```python
from build123d import *

# Parameters (mm, degrees)
BOSS_1_DEPTH    = 5
BOSS_2_DEPTH    = 4.5
S_CYL3_R        = 9.5
BOSS_3_DEPTH    = 3.2
BOSS_4_DEPTH    = 4.5
S_HOLE5_R       = 3.5
HOLE_5_DEPTH    = 4.7
S_HOLE6_R       = 1.7
HOLE_6_DEPTH    = 4.7
S_HOLE7_R       = 1.7
HOLE_7_DEPTH    = 4.7
S_HOLE8_R       = 1.7
HOLE_8_DEPTH    = 4.7
S_HOLE9_R       = 1.7
HOLE_9_DEPTH    = 4.7
S_HOLE10_R      = 3.2
HOLE_10_DEPTH   = 1.6
S_HOLE11_R      = 3.2
HOLE_11_DEPTH   = 1.6
S_HOLE12_R      = 3.2
HOLE_12_DEPTH   = 1.6
S_HOLE13_R      = 3.2
HOLE_13_DEPTH   = 1.6
S_HOLE14_R      = 3.5
HOLE_14_DEPTH   = 7.9
S_HOLE15_R      = 1.7
HOLE_15_DEPTH   = 7.9
S_HOLE16_R      = 1.7
HOLE_16_DEPTH   = 7.9
S_HOLE17_R      = 1.7
HOLE_17_DEPTH   = 7.9
S_HOLE18_R      = 1.7
HOLE_18_DEPTH   = 7.9
S_HOLE19_R      = 3.2
HOLE_19_DEPTH   = 2.1
S_HOLE20_R      = 3.2
HOLE_20_DEPTH   = 2.1
S_HOLE21_R      = 3.2
HOLE_21_DEPTH   = 2.1
S_HOLE22_R      = 3.2
HOLE_22_DEPTH   = 2.1
S_CUT23_W       = 1
S_CUT23_H       = 6.8
POCKET_23_DEPTH = 10
S_HOLE24_R      = 6
HOLE_24_DEPTH   = 5.2
S_HOLE25_R      = 6
HOLE_25_DEPTH   = 5.2
S_HOLE26_R      = 6
HOLE_26_DEPTH   = 5.2
S_CUT27_W       = 1.1
S_CUT27_H       = 4.5
POCKET_27_DEPTH = 16
S_CUT28_W       = 1.1
S_CUT28_H       = 4.5
POCKET_28_DEPTH = 16


with BuildPart() as part:
    # S_prism1 → Boss_1 (new body)
    with BuildSketch(Plane.XY.offset(-33)):
        Polygon((56, -21), (56, 21), (42, 35), (-58, 35), (-68, 25), (-68, -25), (-58, -35), (42, -35), align=None)
    extrude(amount=BOSS_1_DEPTH)

    # S_prism2 → Boss_2 (add)
    with BuildSketch(Plane(origin=(-22, 0, 0), x_dir=(0, 0, -1), z_dir=(1, 0, 0))):
        with BuildLine():
            Line((28.5, -16), (28.5, 16))
            Line((28.5, 16), (-1.0301, 13.8653))
            ThreePointArc((-1.0301, 13.8653), (-9.544808445, 9.785590923), (-13, 0.9989))
            Line((-13, 0.9989), (-13, -0.9989))
            ThreePointArc((-13, -0.9989), (-9.544808445, -9.785590923), (-1.0301, -13.8653))
            Line((-1.0301, -13.8653), (28.5, -16))
        make_face()
    extrude(amount=BOSS_2_DEPTH)



with BuildPart() as body_2:
    # S_cyl3 → Boss_3 (new body)
    with BuildSketch(Plane(origin=(-61.75, 0, 0), x_dir=(0, 0, -1), z_dir=(1, 0, 0))):
        Circle(S_CYL3_R)
    extrude(amount=BOSS_3_DEPTH)


with BuildPart() as part_1:
    add(part.part)

    add(body_2.part)  # Boss_4 merges body 2
    # S_prism4 → Boss_4 (add)
    with BuildSketch(Plane(origin=(-66.25, 0, 0), x_dir=(0, 0, -1), z_dir=(1, 0, 0))):
        with BuildLine():
            Line((28.5, -16), (28.5, 16))
            Line((28.5, 16), (-1.0301, 13.8653))
            ThreePointArc((-1.0301, 13.8653), (-9.544808445, 9.785590923), (-13, 0.9989))
            Line((-13, 0.9989), (-13, -0.9989))
            ThreePointArc((-13, -0.9989), (-9.544808445, -9.785590923), (-1.0301, -13.8653))
            Line((-1.0301, -13.8653), (28.5, -16))
        make_face()
    extrude(amount=BOSS_4_DEPTH)

    # S_hole5 → Hole_5 (cut)
    with BuildSketch(Plane(origin=(-22.1, 0, 0), x_dir=(0, 0, -1), z_dir=(1, 0, 0))):
        Circle(S_HOLE5_R)
    extrude(amount=HOLE_5_DEPTH, mode=Mode.SUBTRACT)

    # S_hole6 → Hole_6 (cut)
    with BuildSketch(Plane(origin=(-22.1, 0, 0), x_dir=(0, 0, -1), z_dir=(1, 0, 0))):
        with Locations((0, 7)):
            Circle(S_HOLE6_R)
    extrude(amount=HOLE_6_DEPTH, mode=Mode.SUBTRACT)

    # S_hole7 → Hole_7 (cut)
    with BuildSketch(Plane(origin=(-22.1, 0, 0), x_dir=(0, 0, -1), z_dir=(1, 0, 0))):
        with Locations((-7, 0)):
            Circle(S_HOLE7_R)
    extrude(amount=HOLE_7_DEPTH, mode=Mode.SUBTRACT)

    # S_hole8 → Hole_8 (cut)
    with BuildSketch(Plane(origin=(-22.1, 0, 0), x_dir=(0, 0, -1), z_dir=(1, 0, 0))):
        with Locations((0, -7)):
            Circle(S_HOLE8_R)
    extrude(amount=HOLE_8_DEPTH, mode=Mode.SUBTRACT)

    # S_hole9 → Hole_9 (cut)
    with BuildSketch(Plane(origin=(-22.1, 0, 0), x_dir=(0, 0, -1), z_dir=(1, 0, 0))):
        with Locations((7, 0)):
            Circle(S_HOLE9_R)
    extrude(amount=HOLE_9_DEPTH, mode=Mode.SUBTRACT)

    # S_hole10 → Hole_10 (cut)
    with BuildSketch(Plane(origin=(-19, 0, 0), x_dir=(0, 0, -1), z_dir=(1, 0, 0))):
        with Locations((0, 7)):
            Circle(S_HOLE10_R)
    extrude(amount=HOLE_10_DEPTH, mode=Mode.SUBTRACT)

    # S_hole11 → Hole_11 (cut)
    with BuildSketch(Plane(origin=(-19, 0, 0), x_dir=(0, 0, -1), z_dir=(1, 0, 0))):
        with Locations((-7, 0)):
            Circle(S_HOLE11_R)
    extrude(amount=HOLE_11_DEPTH, mode=Mode.SUBTRACT)

    # S_hole12 → Hole_12 (cut)
    with BuildSketch(Plane(origin=(-19, 0, 0), x_dir=(0, 0, -1), z_dir=(1, 0, 0))):
        with Locations((0, -7)):
            Circle(S_HOLE12_R)
    extrude(amount=HOLE_12_DEPTH, mode=Mode.SUBTRACT)

    # S_hole13 → Hole_13 (cut)
    with BuildSketch(Plane(origin=(-19, 0, 0), x_dir=(0, 0, -1), z_dir=(1, 0, 0))):
        with Locations((7, 0)):
            Circle(S_HOLE13_R)
    extrude(amount=HOLE_13_DEPTH, mode=Mode.SUBTRACT)

    # S_hole14 → Hole_14 (cut)
    with BuildSketch(Plane(origin=(-66.35, 0, 0), x_dir=(0, 0, -1), z_dir=(1, 0, 0))):
        Circle(S_HOLE14_R)
    extrude(amount=HOLE_14_DEPTH, mode=Mode.SUBTRACT)

    # S_hole15 → Hole_15 (cut)
    with BuildSketch(Plane(origin=(-66.35, 0, 0), x_dir=(0, 0, -1), z_dir=(1, 0, 0))):
        with Locations((0, 7)):
            Circle(S_HOLE15_R)
    extrude(amount=HOLE_15_DEPTH, mode=Mode.SUBTRACT)

    # S_hole16 → Hole_16 (cut)
    with BuildSketch(Plane(origin=(-66.35, 0, 0), x_dir=(0, 0, -1), z_dir=(1, 0, 0))):
        with Locations((-7, 0)):
            Circle(S_HOLE16_R)
    extrude(amount=HOLE_16_DEPTH, mode=Mode.SUBTRACT)

    # S_hole17 → Hole_17 (cut)
    with BuildSketch(Plane(origin=(-66.35, 0, 0), x_dir=(0, 0, -1), z_dir=(1, 0, 0))):
        with Locations((0, -7)):
            Circle(S_HOLE17_R)
    extrude(amount=HOLE_17_DEPTH, mode=Mode.SUBTRACT)

    # S_hole18 → Hole_18 (cut)
    with BuildSketch(Plane(origin=(-66.35, 0, 0), x_dir=(0, 0, -1), z_dir=(1, 0, 0))):
        with Locations((7, 0)):
            Circle(S_HOLE18_R)
    extrude(amount=HOLE_18_DEPTH, mode=Mode.SUBTRACT)

    # S_hole19 → Hole_19 (cut)
    with BuildSketch(Plane(origin=(-66.35, 0, 0), x_dir=(0, 0, -1), z_dir=(1, 0, 0))):
        with Locations((0, 7)):
            Circle(S_HOLE19_R)
    extrude(amount=HOLE_19_DEPTH, mode=Mode.SUBTRACT)

    # S_hole20 → Hole_20 (cut)
    with BuildSketch(Plane(origin=(-66.35, 0, 0), x_dir=(0, 0, -1), z_dir=(1, 0, 0))):
        with Locations((-7, 0)):
            Circle(S_HOLE20_R)
    extrude(amount=HOLE_20_DEPTH, mode=Mode.SUBTRACT)

    # S_hole21 → Hole_21 (cut)
    with BuildSketch(Plane(origin=(-66.35, 0, 0), x_dir=(0, 0, -1), z_dir=(1, 0, 0))):
        with Locations((0, -7)):
            Circle(S_HOLE21_R)
    extrude(amount=HOLE_21_DEPTH, mode=Mode.SUBTRACT)

    # S_hole22 → Hole_22 (cut)
    with BuildSketch(Plane(origin=(-66.35, 0, 0), x_dir=(0, 0, -1), z_dir=(1, 0, 0))):
        with Locations((7, 0)):
            Circle(S_HOLE22_R)
    extrude(amount=HOLE_22_DEPTH, mode=Mode.SUBTRACT)

    # S_cut23 → Pocket_23 (cut)
    with BuildSketch(Plane.XY):
        with Locations((-58.95, 0)):
            Rectangle(S_CUT23_W, S_CUT23_H)
    extrude(amount=POCKET_23_DEPTH, mode=Mode.SUBTRACT)

    # S_hole24 → Hole_24 (cut)
    with BuildSketch(Plane.XY.offset(-33.1)):
        with Locations((-40, 0)):
            Circle(S_HOLE24_R)
    extrude(amount=HOLE_24_DEPTH, mode=Mode.SUBTRACT)

    # S_hole25 → Hole_25 (cut)
    with BuildSketch(Plane.XY.offset(-33.1)):
        with Locations((14, 0)):
            Circle(S_HOLE25_R)
    extrude(amount=HOLE_25_DEPTH, mode=Mode.SUBTRACT)

    # S_hole26 → Hole_26 (cut)
    with BuildSketch(Plane.XY.offset(-33.1)):
        with Locations((36, 0)):
            Circle(S_HOLE26_R)
    extrude(amount=HOLE_26_DEPTH, mode=Mode.SUBTRACT)

    # S_cut27 → Pocket_27 (cut)
    with BuildSketch(Plane.XY.offset(-16)):
        with Locations((-17.95, 14.75)):
            Rectangle(S_CUT27_W, S_CUT27_H)
    extrude(amount=POCKET_27_DEPTH, mode=Mode.SUBTRACT)

    # S_cut28 → Pocket_28 (cut)
    with BuildSketch(Plane.XY.offset(-16)):
        with Locations((-17.95, -14.75)):
            Rectangle(S_CUT28_W, S_CUT28_H)
    extrude(amount=POCKET_28_DEPTH, mode=Mode.SUBTRACT)


solid = part_1.part
```
Part model, mm, in its own coordinate system. A direction names the side the tool comes from. Coordinates: 2 decimals unless noted, no trailing zeros. Loops run counter-clockwise (first coordinate to the right, second up) from the corner with the lowest first, then second, coordinate; pieces in that order, holes last. Notation, with made-up numbers: (-24, 89) - (25, 89) arc R17 cw to (25, 122) - close; hole circle Ø1 at (-28.75, 49). An arc over 180 degrees is marked (long way). Write item = value, one per line. Start each with the question number.
Item 1: Flat gauge pins, fed straight in: pin 1 Ø6.5 at (y, z) = (0, 0) entering from -X; pin 2 Ø1.3 at (y, z) = (14.5, -8.5) entering from +X; pin 3 Ø1.5 at (y, z) = (7, -7.5) entering from -X; pin 4 Ø5.5 at (y, z) = (7, 0) entering from +X. Where does each tip first touch, or does it go through?
Item 2: Wall check: L1, parallel to X at y = -8.5, z = -24; L2, parallel to X at y = 5.5, z = 2.5; L3, parallel to Y at x = -60, z = -1. Give the ranges that are in metal, low to high. Write a range as from..to.
Item 3: Cut at B-B, the plane z = -7. State how many separate pieces and enclosed holes the cut face has, and give its area (3 significant figures).
Item 4: 3-axis set-ups, long thin cutter, end or side, ignore diameter. For faces 1 (the cylindrical face through (-18.26, -3.827, 0.417)), 2 (the flat face through (-17.5, 0, -12)), 3 (the cylindrical face through (31.24, -3.65, -30.54)), 4 (the flat face through (-18.5, -14, -8)), 5 (the flat face through (-64.25, -1.4, -8.4)): which of +Z, -Z, +X, -X, +Y, -Y reach the whole face in a straight line?
Item 5: Cut at A-A, the plane x = -40. Give the cut face in (y, z), and give its area (3 significant figures).
Item 6: Cut at D-D, the plane y = 31. Give the cut face in (x, z), and give its area (3 significant figures).
Item 7: Mould opens along Z. For faces 6 (the flat face through (-68, 0, -31)), 7 (the cylindrical face through (-61.44, 5.34, 0.37)), 8 (the cylindrical face through (-60.172, 2.854, -9.061)), 9 (the flat face through (-64, -14.9, -13.3)) say: released by +Z, released by -Z, zero draft, split by the parting line, or undercut.
Item 8: Cut at C-C, the plane z = -23.5. Give the cut face in (x, y).
The answers:
q1.pin_1 = through
q1.pin_2 = -18.5
q1.pin_3 = -66.25
q1.pin_4 = -19
q2.L1 = -66.25..-61.75, -22..-17.5
q2.L2 = -64.25..-58.55, -22..-19
q2.L3 = -9.45..-8.37, -5.63..-3.35, 3.35..5.63, 8.37..9.45
q3.separate_pieces = 4
q3.enclosed_holes = 0
q3.area = 245 mm2
q4.face_1 = +X
q4.face_2 = +Z, +X, +Y, -Y
q4.face_3 = +Z, -Z
q4.face_4 = +X, -Y
q4.face_5 = -X
q5.outline = (-35, -33) - (-6, -33) - (-6, -28) - (-35, -28) - close; (6, -33) - (35, -33) - (35, -28) - (6, -28) - close
q5.area = 290 mm2
q6.outline = (-62, -33) - (46, -33) - (46, -28) - (-62, -28) - close
q6.area = 540 mm2
q7.face_6 = zero draft
q7.face_7 = undercut
q7.face_8 = undercut
q7.face_9 = released by +Z
q8.outline = (-66.25, -15.64) - (-61.75, -15.64) - (-61.75, 15.64) - (-66.25, 15.64) - close; (-22, -15.64) - (-17.5, -15.64) - (-17.5, 15.64) - (-22, 15.64) - close
